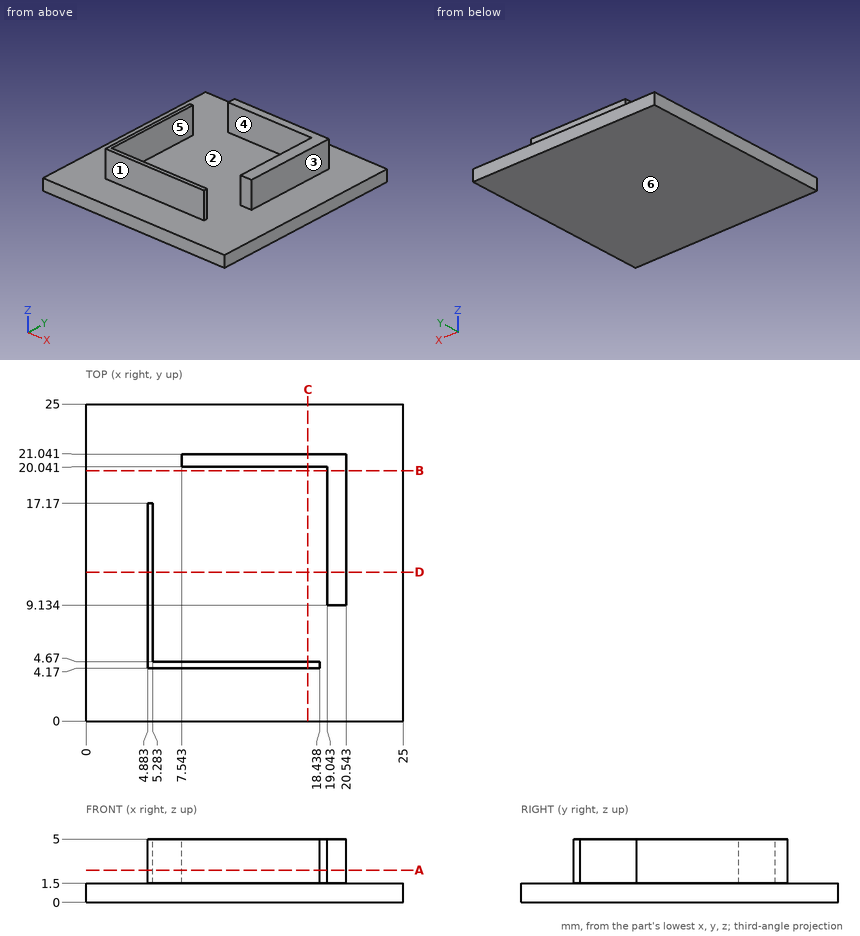
Study the drawing (mm; zero at the part's minimum x, y, z) and answer. A direction names the side the tool comes from. Give positions to 0.01 mm unless a question says otherwise; leave off trailing zeros. Order: outer loops, then holes, each group sorted by start corner. A loop starts at its lowest first (then second) coordinate and runs counter-clockwise, first axis right, second up.
1. Section A-A, the plane z = 2.55 is taken. Determine the outline of the cut face in (x, y).
Result sheet:
outline: (4.88, 4.17) - (18.44, 4.17) - (18.44, 4.67) - (5.28, 4.67) - (5.28, 17.17) - (4.88, 17.17) - close; (7.54, 20.04) - (19.04, 20.04) - (19.04, 9.13) - (20.54, 9.13) - (20.54, 21.04) - (7.54, 21.04) - close
2. Section B-B, the plane y = 19.75 is taken. Determine the outline of the cut face in (x, z).
Result sheet:
outline: (0, 0) - (25, 0) - (25, 1.5) - (20.54, 1.5) - (20.54, 5) - (19.04, 5) - (19.04, 1.5) - (0, 1.5) - close
3. Section D-D, the plane y = 11.75 is taken. Determine the outline of the cut face in (x, z).
Result sheet:
outline: (0, 0) - (25, 0) - (25, 1.5) - (20.54, 1.5) - (20.54, 5) - (19.04, 5) - (19.04, 1.5) - (5.28, 1.5) - (5.28, 5) - (4.88, 5) - (4.88, 1.5) - (0, 1.5) - close
4. Straight lines are drawn through the part: L1, parallel to X at y = 16.25, z = 4.65; L2, parallel to Y at x = 8.75, z = 2.75; L3, parallel to X at y = 9, z = 3.8. For each, find the intervals that lie inside material, in ascending order.
Result sheet:
L1: x = 4.88 to 5.28, 19.04 to 20.54
L2: y = 4.17 to 4.67, 20.04 to 21.04
L3: x = 4.88 to 5.28
5. Each of these flat-tipped pins is pushed along its axis until it touches: P1, Ø0.5, axis at y = 20.5, z = 3.5, coming from the -X side; P2, Ø3, axis at x = 13, z = 4, coming from the +Y side; P3, Ø1, axis at x = 11.5, z = 3, coming from the -Y side. Where does it stop, or does it pass through?
Result sheet:
P1: stops at x = 7.54
P2: stops at y = 21.04
P3: stops at y = 4.17
6. The mould has two halves that part along X. Classify the marked faces 1, 2 and 3: released by +X, released by -X, zero draft, split by the parting line, or undercut.
Result sheet:
face 1: zero draft
face 2: undercut
face 3: released by +X
7. Section C-C, the plane x = 17.5 is taken. Determine the outline of the cut face in (y, z).
Result sheet:
outline: (0, 0) - (25, 0) - (25, 1.5) - (21.04, 1.5) - (21.04, 5) - (20.04, 5) - (20.04, 1.5) - (4.67, 1.5) - (4.67, 5) - (4.17, 5) - (4.17, 1.5) - (0, 1.5) - close
8. For the marked faces 4, 5 and 6, determine the directions among +Z, -Z, +X, -X, +Y, -Y from which every point of the face is accessible in a straight line to the end or side of a thin tool.
Result sheet:
face 4: +Z, -X
face 5: +Z, +Y
face 6: -Z, +X, -X, +Y, -Y
